```python
from build123d import *

# Parameters (mm, degrees)
F1_DEPTH = 50


with BuildPart() as f1:
    # F0 (on Front) → F1 (new body)
    with BuildSketch(Plane.XZ):
        Polygon((-13.242977, 0), (0, 0), (0, 14.5), (-3, 14.5), (-3, 17.5), (0, 17.5), (0, 32), (-3, 32), (-14.805269, 20.194731), (-14.805269, 17.5), (-16.805269, 17.5), (-18.805269, 17.5), (-18.805269, 20.323527), (-29.687413, 31.906461), (-32.685954, 32), (-32.685954, 17.5), (-29.685954, 17.5), (-29.685954, 14.5), (-32.685954, 14.5), (-32.685954, 0), (-19.442977, 0), (-19.442977, 4.2), (-22.442977, 4.2), (-22.442977, 7.2), (-10.242977, 7.2), (-10.242977, 4.2), (-13.242977, 4.2), align=None)
    extrude(amount=F1_DEPTH)


solid = f1.part
```
Verification items for the finished model (mm, model axes). A direction names the side the tool comes from. Coordinates: 2 decimals unless noted, no trailing zeros. Loops run counter-clockwise (first coordinate to the right, second up) from the corner with the lowest first, then second, coordinate; pieces in that order, holes last. Notation, with made-up numbers: (-37.75, 51.5) - (-17.75, 51.5) arc R16 cw to (-17.75, 67.5) - close; hole circle Ø5 at (-2, -15). An arc over 180 degrees is marked (long way). Return JSON: item names as keys, results as strings.
1. Section check B-B, the plane y = -41. Record the boundary of the cut face in (x, z), then the cut area to 3 significant figures.
Established:
{"outline": "(-32.69, 0) - (-19.44, 0) - (-19.44, 4.2) - (-22.44, 4.2) - (-22.44, 7.2) - (-10.24, 7.2) - (-10.24, 4.2) - (-13.24, 4.2) - (-13.24, 0) - (0, 0) - (0, 14.5) - (-3, 14.5) - (-3, 17.5) - (0, 17.5) - (0, 32) - (-3, 32) - (-14.81, 20.19) - (-14.81, 17.5) - (-18.81, 17.5) - (-18.81, 20.32) - (-29.69, 31.91) - (-32.69, 32) - (-32.69, 17.5) - (-29.69, 17.5) - (-29.69, 14.5) - (-32.69, 14.5) - close", "area": "773 mm2"}
2. Section check C-C, the plane x = -21.5. Record the boundary of the cut face in (y, z).
Established:
{"outline": "(-50, 0) - (0, 0) - (0, 4.2) - (-50, 4.2) - close; (-50, 7.2) - (0, 7.2) - (0, 23.19) - (-50, 23.19) - close"}
3. Section check D-D, the plane x = -4.5. Record the boundary of the cut face in (y, z), then the cut area to 4 significant figures.
Established:
{"outline": "(-50, 0) - (0, 0) - (0, 30.5) - (-50, 30.5) - close", "area": "1,525 mm2"}
4. Tool access check on faces 1 (the flat face through (-3, -25, 16)), 2 (the flat face through (-21, -25, 4.2)), 3 (the flat face through (-19.443, -25, 2)), 4 (the flat face through (-24.17, -24.65, 26.034)). Record the directions out of +Z, -Z, +X, -X, +Y, -Y that give a thin tool (end or side, any length) a straight path to the whole face; none if there is none.
Established:
{"face 1": "+X, +Y, -Y", "face 2": "+Y, -Y", "face 3": "-Z, +Y, -Y", "face 4": "+Z, +Y, -Y"}
5. Thickness scan on L1, parallel to X at y = -1.5, z = 19.5; L2, parallel to X at y = -26, z = 4; L3, parallel to Z at x = -22, y = -40.5. Record the ranges inside material, lowest first.
Established:
{"L1": "x = -32.69 to -18.81, -14.81 to 0", "L2": "x = -32.69 to -19.44, -13.24 to 0", "L3": "z = 0 to 4.2, 7.2 to 23.72"}
6. Section check A-A, the plane z = 6. Record the boundary of the cut face in (x, y), then the cut area to 3 significant figures.
Established:
{"outline": "(-32.69, -50) - (-22.44, -50) - (-22.44, 0) - (-32.69, 0) - close; (-10.24, -50) - (0, -50) - (0, 0) - (-10.24, 0) - close", "area": "1,020 mm2"}
7. Go/stop test with flat-tipped pins: pin 1 (3.5 mm diameter, centred on x = -11.5, y = -32, fed in from +Z); pin 2 (5 mm diameter, centred on x = -13, y = -23.5, fed in from +Z); pin 3 (6 mm diameter, centred on x = -8, y = -24, fed in from +Z). Record where each tip stops, or that it passes through.
Established:
{"pin 1": "stops at z = 25.25", "pin 2": "stops at z = 24.5", "pin 3": "stops at z = 30"}
